Part model, mm, in its own coordinate system. A direction names the side the tool comes from. Give positions to 0.01 mm unless a question says otherwise; leave off trailing zeros. Order: outer loops, then holes, each group sorted by start corner. A loop starts at its lowest first (then second) coordinate and runs counter-clockwise, first axis right, second up. Notation, with made-up numbers: (49, -30) -> (96, -30) arc R17 cw to (96, -19) -> close; hole circle Ø9 at (-23.5, 60.5). An arc over 180 degrees is marked (long way). Write item = value, one per line. Start each with the question number.
Item 1: Band-saw the part on A-A on z = -101.6. Write the cut outline in (x, y), plus the area to 3 significant figures.
Item 2: Pull direction X, two halves, no side cores. Call faces 1 (the face through (-149, 15, -107)), 2 (the face through (-164.997, 7.395, -101.336)), 3 (the face through (164.997, 7.395, -101.864)), 4 (the face through (109.85, 3.94, -101.66)): +X half, -X half, draft (parallel to the pull), parting line (faces both ways), or undercut.
Item 3: Band-saw the part on C-C on x = -126.5. Write the cut outline in (y, z).
Item 4: Drill centre lines: line 1 along X through (y, z) = (4, -101) (3 decimals); line 2 along X through (y, z) = (11.5, -107); line 3 along X through (y, z) = (12.25, -110). Where is each one in solid material? Low to high.
Item 5: Flat gauge pins, fed straight in: P1, Ø1, axis at x = 100, z = -111, coming from the +Y side; P2, Ø3, axis at y = 9, z = -104, coming from the +X side; P3, Ø1.5, axis at y = 7.5, z = -106, coming from the +X side. Where does each tip first touch, or does it go through?
Item 6: Band-saw the part on B-B on y = 3.75. Write the cut outline in (x, z), plus the area to 3 significant figures.
Item 7: Tool access for faces 5 (the face through (-109.85, 3.94, -101.54)), 6 (the face through (77.306, 11.549, -101.432)), 7 (the face through (149, 15, -107)): list every direction of +Z, -Z, +X, -X, +Y, -Y with a clear straight run to the whole face (end or side of a thin tool).
```python
from build123d import *

# Parameters (mm, degrees)
BOSS_EXTRUDE2_DEPTH = 15
CUT_EXTRUDE3_DEPTH  = 168.40967714


with BuildPart() as part:
    # Sketch1 → Boss-Extrude2 (new body)
    with BuildSketch(Plane(origin=(0, 0, 0), x_dir=(1, 0, 0), z_dir=(0, 1, 0))):
        with BuildLine():
            Line((-153, 113.6), (153, 113.6))
            ThreePointArc((153, 113.6), (165, 101.6), (153, 89.6))
            Line((153, 89.6), (-153, 89.6))
            ThreePointArc((-153, 89.6), (-165, 101.6), (-153, 113.6))
        make_face()
        with BuildLine():
            Line((-153, 104.35), (-142, 104.35))
            ThreePointArc((-142, 104.35), (-139.25, 101.6), (-142, 98.85))
            Line((-142, 98.85), (-153, 98.85))
            ThreePointArc((-153, 98.85), (-155.75, 101.6), (-153, 104.35))
        make_face(mode=Mode.SUBTRACT)
        with BuildLine():
            Line((-107.1, 104.35), (-96.1, 104.35))
            ThreePointArc((-96.1, 104.35), (-93.35, 101.6), (-96.1, 98.85))
            Line((-96.1, 98.85), (-107.1, 98.85))
            ThreePointArc((-107.1, 98.85), (-109.85, 101.6), (-107.1, 104.35))
        make_face(mode=Mode.SUBTRACT)
        with BuildLine():
            Line((96.1, 104.35), (107.1, 104.35))
            ThreePointArc((107.1, 104.35), (109.85, 101.6), (107.1, 98.85))
            Line((107.1, 98.85), (96.1, 98.85))
            ThreePointArc((96.1, 98.85), (93.35, 101.6), (96.1, 104.35))
        make_face(mode=Mode.SUBTRACT)
        with BuildLine():
            Line((153, 98.85), (142, 98.85))
            ThreePointArc((142, 98.85), (139.25, 101.6), (142, 104.35))
            Line((142, 104.35), (153, 104.35))
            ThreePointArc((153, 104.35), (155.75, 101.6), (153, 98.85))
        make_face(mode=Mode.SUBTRACT)
    extrude(amount=BOSS_EXTRUDE2_DEPTH)

    # Sketch4 → Cut-Extrude3 (cut, through all)
    with BuildSketch(Plane.XY.offset(-89.6)):
        Polygon((-132.5, 15), (-119.1, 8), (-84.1, 8), (-70.7, 15), align=None)
        Polygon((119.1, 8), (132.5, 15), (70.7, 15), (84.1, 8), align=None)
    extrude(amount=-CUT_EXTRUDE3_DEPTH, mode=Mode.SUBTRACT)


solid = part.part
```
Values found:
q1.outline = (-165, 0) -> (-155.75, 0) -> (-155.75, 15) -> (-165, 15) -> close; (-139.25, 0) -> (-109.85, 0) -> (-109.85, 8) -> (-119.1, 8) -> (-132.5, 15) -> (-139.25, 15) -> close; (-93.35, 0) -> (93.35, 0) -> (93.35, 8) -> (84.1, 8) -> (70.7, 15) -> (-70.7, 15) -> (-84.1, 8) -> (-93.35, 8) -> close; (109.85, 0) -> (139.25, 0) -> (139.25, 15) -> (132.5, 15) -> (119.1, 8) -> (109.85, 8) -> close; (155.75, 0) -> (165, 0) -> (165, 15) -> (155.75, 15) -> close
q1.area = 3,510 mm^2
q2.face_1 = draft
q2.face_2 = -X half
q2.face_3 = +X half
q2.face_4 = undercut
q3.outline = (0, -113.6) -> (11.87, -113.6) -> (11.87, -89.6) -> (0, -89.6) -> close
q4.line_1 = -164.985 to -155.684, -139.316 to -109.784, -93.416 to 93.416, 109.784 to 139.316, 155.684 to 164.985
q4.line_2 = -163.72 to -125.8, -77.4 to 77.4, 125.8 to 163.72
q4.line_3 = -161.57 to -127.24, -75.96 to 75.96, 127.24 to 161.57
q5.P1 = 8
q5.P2 = 164.97
q5.P3 = 164.43
q6.outline = (-153, -113.6) -> (153, -113.6) arc R12 ccw to (153, -89.6) -> (-153, -89.6) arc R12 ccw to start; hole (-153, -104.35) -> (-142, -104.35) arc R2.75 ccw to (-142, -98.85) -> (-153, -98.85) arc R2.75 ccw to start; hole (-107.1, -104.35) -> (-96.1, -104.35) arc R2.75 ccw to (-96.1, -98.85) -> (-107.1, -98.85) arc R2.75 ccw to start; hole (96.1, -104.35) -> (107.1, -104.35) arc R2.75 ccw to (107.1, -98.85) -> (96.1, -98.85) arc R2.75 ccw to start; hole (142, -104.35) -> (153, -104.35) arc R2.75 ccw to (153, -98.85) -> (142, -98.85) arc R2.75 ccw to start
q6.area = 7,460 mm^2
q7.face_5 = +Y, -Y
q7.face_6 = +Z, -Z, +Y
q7.face_7 = +Z, -Z, +X, -X, +Y
